Read the model definition and answer for the solid it produces. Units are mm, in the model's axes. A direction names the side the tool comes from. Round coordinates to 2 decimals unless told otherwise and drop trailing zeros. Order: outer loops, then holes, each group sorted by start corner. A loop starts at its lowest first (then second) coordinate and runs counter-clockwise, first axis right, second up. Notation, with made-up numbers: (-28, 87.5) - (1, 87.5) arc R10 ccw to (1, 100.5) - close; hole circle Ø4 at (-37.5, -15.5). An arc over 180 degrees is marked (long way). Answer as a JSON object with one key per item and string values. Group by question number.
Q1. A cutting plane is placed at A-A on z = 11.5. Determine the outline of the cut face in (x, y).
Q2. The mould has two halves that part along X. Classify faces 4 (the cylindrical face through (45.174, 50.036, 6.439)), 5 (the cylindrical face through (64.224, 22.354, 6.439)), 6 (the flat face through (48, 0, 6)): pulls with the +X half, pulls with the -X half, needs draft (parallel to the pull), parting line crosses it, or undercut.
Q3. Consider line 1 (X direction, y = 36.5, z = 8.5); line 2 (Y direction, x = 39.5, z = 0.5); line 3 (Y direction, x = 88, z = 11). Determine where each line is inside the solid, lowest interval first.
Q4. A tool of negligible diameter and unlimited length cuts with its end or side. For faces 1 (the flat face through (79, 21.59, 6)), 2 (the flat face through (13, 50.8, 6)), 3 (the flat face through (25.4, 38, 6)), from which of +Z, -Z, +X, -X, +Y, -Y can it reach the whole face along a straight path? Write none if from no direction.
Q5. A cutting plane is placed at C-C on x = 32. Determine the outline of the cut face in (y, z), and give its area (3 significant figures).
Q6. Given pin 1 Ø2 at (x, z) = (61, 6) entering from -Y; pin 2 Ø4 at (y, z) = (40.5, 4.5) entering from +X, each flat-ended and moving along its own axis, determine where each tip first touches the part or whether it passes through.
Q7. A cutting plane is placed at B-B on x = 77. Determine the outline of the cut face in (y, z).
```python
from build123d import *

# Parameters (mm, degrees)
BOSS_EXTRUDE1_DEPTH = 12.7
FILLET1_R           = 2.54


with BuildPart() as part:
    # Sketch1 → Boss-Extrude1 (new body)
    with BuildSketch(Plane.XY):
        Polygon((0, 0), (0, 50.8), (25.4, 50.8), (25.4, 25.4), (44.45, 25.4), (44.45, 50.8), (63.5, 50.8), (63.5, 21.59), (95.25, 21.59), (95.25, 0), align=None)
    extrude(amount=BOSS_EXTRUDE1_DEPTH)

    # Fillet1
    fillet1_edges = [part.edges().sort_by_distance(p)[0] for p in [
        (0, 50.8, 6.35),
        (25.4, 50.8, 6.35),
        (25.4, 25.4, 6.35),
        (44.45, 25.4, 6.35),
        (44.45, 50.8, 6.35),
        (63.5, 50.8, 6.35),
        (63.5, 21.59, 6.35),
        (95.25, 21.59, 6.35),
    ]]
    fillet(fillet1_edges, radius=FILLET1_R)


solid = part.part
```
Result set:
{
 "1": {"outline": "(0, 0) - (95.25, 0) - (95.25, 19.05) arc R2.54 ccw to (92.71, 21.59) - (66.04, 21.59) arc R2.54 cw to (63.5, 24.13) - (63.5, 48.26) arc R2.54 ccw to (60.96, 50.8) - (46.99, 50.8) arc R2.54 ccw to (44.45, 48.26) - (44.45, 27.94) arc R2.54 cw to (41.91, 25.4) - (27.94, 25.4) arc R2.54 cw to (25.4, 27.94) - (25.4, 48.26) arc R2.54 ccw to (22.86, 50.8) - (2.54, 50.8) arc R2.54 ccw to (0, 48.26) - close"},
 "2": {"face 4": "undercut", "face 5": "pulls with the +X half", "face 6": "needs draft"},
 "3": {"line 1": "x = 0 to 25.4, 44.45 to 63.5", "line 2": "y = 0 to 25.4", "line 3": "y = 0 to 21.59"},
 "4": {"face 1": "+Z, -Z, +X, +Y", "face 2": "+Z, -Z, +X, -X, +Y", "face 3": "+Z, -Z, +Y"},
 "5": {"outline": "(0, 0) - (25.4, 0) - (25.4, 12.7) - (0, 12.7) - close", "area": "323 mm²"},
 "6": {"pin 1": "stops at y = 0", "pin 2": "stops at x = 63.5"},
 "7": {"outline": "(0, 0) - (21.59, 0) - (21.59, 12.7) - (0, 12.7) - close"}
}
